The listing builds one solid part. Answer for the finished solid, in the listing's coordinates (mm). A direction names the side the tool comes from. Coordinates: 2 decimals unless noted, no trailing zeros. Write each loop counter-clockwise with the first axis right and the second up, starting at its lowest first coordinate (ties: lowest second). Pieces come first, ordered by that corner, then holes.
from build123d import *

# Parameters (mm, degrees)
F0_W        = 140
F0_H        = 252.5
F0_R        = 1
F0_W_2      = 94
F0_H_2      = 152.5
F0_R_2      = 2.5
F0_W_3      = 12
F0_H_3      = 34
F1_DEPTH    = 15.56
F2_DEPTH    = 10.56
F3_T1_DEPTH = 165.7168298797
F3_T3_DEPTH = 278.2168298797
F4_SIZE     = 2.5
F5_R        = 3
F6_DEPTH    = 10
F7_SIZE     = 4.99999


# Not quite as in the source:
# - a fillet or chamfer that OpenCascade refuses, or shapes differently, is made with other operations: its cross-section is extruded or revolved along the edge and cut away or added
# - a fillet or chamfer is up to 0.001 mm smaller than in the source, because OpenCascade refuses the exact size
# - a feature names something its author has since deleted; it is built from what else it names


with BuildPart() as f1:
    # F0 (on Front) → F1 (new body)
    with BuildSketch(Plane.XZ):
        with Locations((-70, 126.25)):
            Rectangle(F0_W, F0_H)
        with Locations((-135, 5)):
            Circle(F0_R, mode=Mode.SUBTRACT)
        with Locations((-5, 5)):
            Circle(F0_R, mode=Mode.SUBTRACT)
        with Locations((-135, 247.5)):
            Circle(F0_R, mode=Mode.SUBTRACT)
        Polygon((-130, 44), (-130, 242.5), (-10, 242.5), (-10, 44), (-64, 44), (-64, 10), (-76, 10), (-76, 44), align=None, mode=Mode.SUBTRACT)
        with Locations((-5, 247.5)):
            Circle(F0_R, mode=Mode.SUBTRACT)
        Polygon((-10, 242.5), (-130, 242.5), (-130, 44), (-76, 44), (-64, 44), (-10, 44), align=None)
        with Locations((-70, 143.25)):
            Rectangle(F0_W_2, F0_H_2, mode=Mode.SUBTRACT)
        with Locations((-70, 232.5)):
            Circle(F0_R_2, mode=Mode.SUBTRACT)
        with Locations((-70, 27)):
            Rectangle(F0_W_3, F0_H_3)
    extrude(amount=F1_DEPTH)

    # F0 (on Front) → F2 (cut)
    with BuildSketch(Plane.XZ):
        Polygon((-10, 242.5), (-130, 242.5), (-130, 44), (-76, 44), (-64, 44), (-10, 44), align=None)
        with Locations((-70, 143.25)):
            Rectangle(F0_W_2, F0_H_2, mode=Mode.SUBTRACT)
        with Locations((-70, 232.5)):
            Circle(F0_R_2, mode=Mode.SUBTRACT)
        with Locations((-70, 27)):
            Rectangle(F0_W_3, F0_H_3)
    extrude(amount=F2_DEPTH, mode=Mode.SUBTRACT)

    # F3: chamfer of 5 on 4 edges, made by hand

    # F3_s2 → F3_t1 (cut)
    with BuildSketch(Plane.YZ.offset(-152.8584149398)):
        Polygon((-10.56, 0), (-15.56, 5), (-15.56, 0), align=None)
        Polygon((-15.56, 247.5), (-10.56, 252.5), (-15.56, 252.5), align=None)
    extrude(amount=F3_T1_DEPTH, mode=Mode.SUBTRACT)

    # F3_s4 → F3_t3 (cut)
    with BuildSketch(Plane.XY.offset(-12.8584149398)):
        Polygon((-140, -10.56), (-135, -15.56), (-140, -15.56), align=None)
        Polygon((0, -10.56), (-5, -15.56), (0, -15.56), align=None)
    extrude(amount=F3_T3_DEPTH, mode=Mode.SUBTRACT)

    # F4
    f4_edges = [f1.edges().sort_by_distance(p)[0] for p in [
        (-72.5, -15.56, 232.5),
    ]]
    chamfer(f4_edges, length=F4_SIZE)

    # F5 (on face) → F6 (cut)
    with BuildSketch(Plane.XZ.offset(15.56)):
        with Locations((-135, 247.5)):
            Circle(F5_R)
        with Locations((-135, 5)):
            Circle(F5_R)
        with Locations((-5, 247.5)):
            Circle(F5_R)
        with Locations((-5, 5)):
            Circle(F5_R)
    extrude(amount=-F6_DEPTH, mode=Mode.SUBTRACT)

    # F7 (size 5 in the source; OpenCascade refuses exactly that, so slightly less here)
    f7_edges = [f1.edges().sort_by_distance(p)[0] for p in [
        (-70, -15.56, 67),
        (-117, -15.56, 143.25),
        (-23, -15.56, 143.25),
        (-70, -15.56, 219.5),
    ]]
    chamfer(f7_edges, length=F7_SIZE)


solid = f1.part
1. For a pull along Z with two mould halves and no side action, classify faces 4 (the flat face through (-71, -5, 252.5)), 5 (the flat face through (-6, -5.56, 6)), 6 (the flat face through (-2.46, -13.02, 124.48)) as pulls with the +Z half, pulls with the -Z half, needs draft (parallel to the pull), parting line crosses it, or undercut.
Results found:
face 4: pulls with the +Z half
face 5: undercut
face 6: needs draft
2. A tool of negligible diameter and unlimited length cuts with its end or side. For faces 1 (the flat face through (-140, -5, 124)), 2 (the flat face through (-3.7, -5.56, 247.5)), 3 (the flat face through (-10, -5, 142)), from which of +Z, -Z, +X, -X, +Y, -Y can it reach the whole face along a straight path? Write none if from no direction.
Results found:
face 1: +Z, -Z, -X, +Y, -Y
face 2: -Y
face 3: +Y
3. Flat-ended cylindrical pins translate along their axes: P1, Ø6, axis at x = -70, z = 232.5, coming from the +Y side; P2, Ø5.5, axis at x = -5, z = 5, coming from the -Y side; P3, Ø1, axis at y = -13, z = 59.5, coming from the +X side; P4, Ø1.6, axis at x = -135, z = 5, coming from the +Y side. Find the tip coordinate at first contact, or state that the pin passes through.
Results found:
P1: stops at y = -10.56
P2: stops at y = -5.56
P3: stops at x = -1.94
P4: passes through
4. Section A-A on z = 232.5 is taken. Give the vertices of the cut face in (x, y).
Results found:
outline: (-140, -10.56) - (-135, -15.56) - (-75, -15.56) - (-72.5, -13.06) - (-72.5, -10.56) - (-130, -10.56) - (-130, 0) - (-140, 0) - close; (-67.5, -13.06) - (-65, -15.56) - (-5, -15.56) - (0, -10.56) - (0, 0) - (-10, 0) - (-10, -10.56) - (-67.5, -10.56) - close
5. Section B-B on x = -70 is taken. State how many separate pieces and enclosed holes the cut face has, then the cut area to 3 significant figures.
Results found:
separate pieces: 3
enclosed holes: 0
area: 630 mm2
6. Find the intervals of material crossed by L1, parallel to Z at x = -5, y = -10; L2, parallel to X at y = -3.1, z = 247.5; L3, parallel to X at y = -10, z = 247.5, in increasing order.
Results found:
L1: z = 0 to 2, 8 to 244.5, 250.5 to 252.5
L2: x = -140 to -136, -134 to -6, -4 to 0
L3: x = -140 to -138, -132 to -8, -2 to 0
